Geometry: final body of the model. Coordinates: model frame, mm. Face numbers are marked on the shaded views. A direction names the side the tool comes from. Give positions to 0.01 mm unless a question says otherwise; leave off trailing zeros. Loops run counter-clockwise (first coordinate to the right, second up) from the corner with the lowest first, then second, coordinate; pieces in that order, holes last. Notation, with made-up numbers: (4.5, 45) - (8.5, 45) arc R24 cw to (8.5, 58) - close; hole circle Ø4 at (54.25, -4). An arc over 180 degrees is marked (long way). Answer in a Markdown table with one row per item.
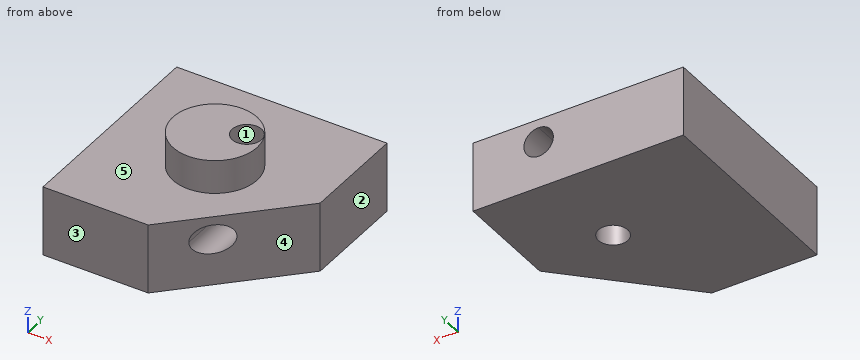
from build123d import *

# Parameters (mm, degrees)
F0_W     = 25
F0_H     = 25
F1_DEPTH = 8.3
F2_R     = 5
F3_DEPTH = 4
F5_DEPTH = 25
F6_R     = 1.75
F7_DEPTH = 25
F9_DEPTH = 25


with BuildPart() as f1:
    # F0 (on Top) → F1 (new body)
    with BuildSketch(Plane.XY):
        Rectangle(F0_W, F0_H)
    extrude(amount=F1_DEPTH)

    # F2 (on face) → F3 (join)
    with BuildSketch(Plane.XY.offset(8.3)):
        Circle(F2_R)
    extrude(amount=F3_DEPTH)

    # F4 (on face) → F5 (cut)
    with BuildSketch(Plane.XY.offset(8.3)):
        Polygon((12.5, -12.5), (12.5, 0), (0, -12.5), align=None)
    extrude(amount=-F5_DEPTH, mode=Mode.SUBTRACT)

    # F6 (on face) → F7 (cut)
    with BuildSketch(Plane.XY.offset(12.3)):
        with Locations((2.900001, 1.400001)):
            Circle(F6_R)
    extrude(amount=-F7_DEPTH, mode=Mode.SUBTRACT)

    # F8 (on face) → F9 (cut)
    with BuildSketch(Plane(origin=(0, 12.5, 0), x_dir=(-1, 0, 0), z_dir=(0, 1, 0))):
        with BuildLine():
            ThreePointArc((-4.7, 7.3), (-5.937437, 4.312563), (-2.95, 5.55))
            ThreePointArc((-2.95, 5.55), (-3.462563, 6.787437), (-4.7, 7.3))
        make_face()
    extrude(amount=-F9_DEPTH, mode=Mode.SUBTRACT)


solid = f1.part
Q1. Cut plane B-B (y = 8). Output: boundary loops of the cut face in (x, z), and give its area (3 significant figures).
Check values:
| item | result |
|---|---|
| outline | (-12.5, 0) - (12.5, 0) - (12.5, 8.3) - (-12.5, 8.3) - close; hole circle Ø3.5 at (4.7, 5.55) |
| area | 198 mm² |
Q2. Reachability of the marked faces 4 and 5 from +Z, -Z, +X, -X, +Y, -Y: full face, straight path, thin tool, end or side. Return the list, or none.
Check values:
| item | result |
|---|---|
| face 4 | +Z, -Z, +X, -Y |
| face 5 | +Z |
Q3. First-contact query: pin 1 (5 mm diameter, centred on x = -6, y = 9.5, fed in from +Z); pin 2 (3 mm diameter, centred on x = -2.5, y = -5.5, fed in from -Z); pin 3 (2 mm diameter, centred on y = -8.5, z = 10, fed in from +X); pin 4 (5.5 mm diameter, centred on x = 4.7, z = 5.55, fed in from -Y). Flat tips, straight axial feed; report the tip coordinate or a pass-through.
Check values:
| item | result |
|---|---|
| pin 1 | z = 8.3 |
| pin 2 | z = 0 |
| pin 3 | through |
| pin 4 | y = -10.55 |
Q4. Cut plane A-A (z = 5.25). Output: boundary loops of the cut face in (x, y), and give its area (3 significant figures).
Check values:
| item | result |
|---|---|
| outline | (-12.5, -12.5) - (0, -12.5) - (2.98, -9.52) - (2.98, -0.35) arc R1.75 cw (long way) to (2.98, 3.15) - (2.98, 12.5) - (-12.5, 12.5) - close; (6.42, -6.08) - (12.5, 0) - (12.5, 12.5) - (6.42, 12.5) - close |
| area | 472 mm² |
Q5. Material intervals for line 1 along X through (y, z) = (7, 5.55); line 2 along Z through (x, y) = (4.7, 5.75); line 3 along Z through (x, y) = (4.7, 1.5), sorted ascending.
Check values:
| item | result |
|---|---|
| line 1 | -12.5 to 2.95, 6.45 to 12.5 |
| line 2 | 0 to 3.8, 7.3 to 8.3 |
| line 3 | 0 to 3.8, 7.3 to 12.3 |
Q6. Cut plane C-C (y = -6.75). Output: boundary loops of the cut face in (x, z), and give its area (3 significant figures).
Check values:
| item | result |
|---|---|
| outline | (-12.5, 0) - (5.75, 0) - (5.75, 4.15) arc R1.75 cw (long way) to (5.75, 6.95) - (5.75, 8.3) - (-12.5, 8.3) - close |
| area | 143 mm² |
Q7. Draft query along Y for the marked faces 1, 2 and 3. Return one class per face: pulls with the +Y half, pulls with the -Y half, needs draft (parallel to the pull), parting line crosses it, or undercut.
Check values:
| item | result |
|---|---|
| face 1 | undercut |
| face 2 | needs draft |
| face 3 | pulls with the -Y half |
